Input: part model. Units: mm. Frame: model coordinates. A direction names the side the tool comes from. Coordinates: 2 decimals unless noted, no trailing zeros. Write each loop counter-clockwise with the first axis right and the second up, starting at its lowest first coordinate (ties: lowest second). Pieces come first, ordered by that corner, then holes. Notation, with made-up numbers: M 64.25,67 L 109.25,67 A29 cw 109.25,90 Z; hole C 23.25,74 d9. An arc over 180 degrees is marked long. Write each question's results on one line, items separated by ' | '. Start each with the question number.
1. Pull-direction query (Y, two-part tool) for faces 1 (the flat face through (0.9, -2, 6)), 2 (the flat face through (-1.965, -3.34, -8.381)), 3 (the flat face through (-3.875, 0, -8)); classes: +Y half, -Y half, draft (parallel to the pull), parting line (faces both ways), or undercut.
2. Set-up query: faces 4 (the flat face through (1.91, -3.37, -8.38)), 5 (the cylindrical face through (1.565, -13.017, 6.246)), 6 (the flat face through (2.4, 0, 6)), 7 (the flat face through (-1.91, 3.37, -8.38)). Return all of +Z, -Z, +X, -X, +Y, -Y with unobstructed straight access to the full face (end or side cutting, diameter ignored); none if empty.
3. Section query A-A, the plane y = 0. Output: boundary loops of the cut face in (x, z) (3 decimals).
4. Section query C-C, the plane z = 0.5. Output: boundary loops of the cut face in (x, y), and give its area (3 significant figures).
5. Ray query, probe 1 along Z at (x, y) = (-7, 8.5); probe 2 along Z at (x, y) = (1, 4); probe 3 along X at (y, z) = (0.5, -15) (3 decimals). Return the intervals inside material, ascending.
6. First-contact query: pin 1 (6 mm diameter, centred on x = 11, y = 15.5, fed in from -Z); pin 2 (1.7 mm diameter, centred on y = 1.5, z = 6.5, fed in from +X); pin 3 (10 mm diameter, centred on y = 5, z = -5.5, fed in from -X) (3 decimals). Flat tips, straight axial feed; report the tip coordinate or a pass-through.
7. Section query B-B, the plane z = -11.5. Output: boundary loops of the cut face in (x, y) (3 decimals), and give its area (3 significant figures).
```python
from build123d import *

# Parameters (mm, degrees)
F1_DEPTH  = 17
F2_R      = 4.7
F3_DEPTH  = 6
F4_R      = 19.4
F5_DEPTH  = 3
F6_R      = 1
F7_W      = 1.5
F7_H      = 1.8
F7_W_2    = 1.8
F7_H_2    = 1.5
F8_DEPTH  = 6
F10_DEPTH = 0.5


with BuildPart() as f1:
    # F0 (on Top) → F1 (new body)
    with BuildSketch(Plane.XY):
        Polygon((3.875, -2.2372322931), (3.875, 2.2372322931), (0, 4.4744645862), (-3.875, 2.2372322931), (-3.875, -2.2372322931), (0, -4.4744645862), align=None)
    extrude(amount=-F1_DEPTH)

    # F2 (on face) → F3 (join)
    with BuildSketch(Plane.XY):
        Circle(F2_R)
    extrude(amount=F3_DEPTH)

    # F4 (on face) → F5 (join)
    with BuildSketch(Plane.XY.offset(6)):
        Circle(F4_R)
    extrude(amount=F5_DEPTH)

    # F6
    f6_edges = [f1.edges().sort_by_distance(p)[0] for p in [
        (-19.4, 0, 6),
        (-19.4, 0, 9),
    ]]
    fillet(f6_edges, radius=F6_R)

    # F7 (on face) → F8 (cut)
    with BuildSketch(Plane.XY.offset(9)):
        with Locations((-1.65, 0.05)):
            Rectangle(F7_W, F7_H)
        with Locations((0, 1.7)):
            Rectangle(F7_W_2, F7_H_2)
        with Locations((0, 0.05)):
            Rectangle(F7_W_2, F7_H)
        with Locations((1.65, 0.05)):
            Rectangle(F7_W, F7_H)
        with Locations((0, -1.6)):
            Rectangle(F7_W_2, F7_H_2)
    extrude(amount=-F8_DEPTH, mode=Mode.SUBTRACT)

    # F9 (on face) → F10 (cut)
    with BuildSketch(Plane(origin=(0, 0, 6), x_dir=(1, 0, 0), z_dir=(0, 0, -1))):
        with BuildLine():
            Line((0.12, 16.1495609697), (0.12, 16.3995609697))
            ThreePointArc((0.12, 16.3995609697), (-1.8790989856, 14.4595880123), (0, 12.4031642156))
            Line((0, 12.4031642156), (0, 12.6536801032))
            ThreePointArc((0, 12.6536801032), (-1.6289699135, 14.4595963078), (0.12, 16.1495609697))
        make_face()
        with BuildLine():
            Line((0, 12.6536801032), (0, 12.4031642156))
            ThreePointArc((0, 12.4031642156), (0.1250097944, 12.3995672443), (0.25, 12.4037904418))
            Line((0.25, 12.4037904418), (0.25, 12.6543962211))
            ThreePointArc((0.25, 12.6543962211), (0.1250128042, 12.6495681492), (0, 12.6536801032))
        make_face()
        with BuildLine():
            ThreePointArc((0.25, 12.4037904418), (0.1250097944, 12.3995672443), (0, 12.4031642156))
            Line((0, 12.4031642156), (0, 10.8995609697))
            Line((0, 10.8995609697), (0.25, 10.8995609697))
            Line((0.25, 10.8995609697), (0.25, 12.4037904418))
        make_face()
        with BuildLine():
            Line((0.25, 12.6543962211), (0.25, 12.4037904418))
            ThreePointArc((0.25, 12.4037904418), (1.5794519519, 13.0320815366), (2.12, 14.3995609697))
            Line((2.12, 14.3995609697), (1.87, 14.3995609697))
            ThreePointArc((1.87, 14.3995609697), (1.865506934, 14.2742392103), (1.8520508076, 14.1495609697))
            ThreePointArc((1.8520508076, 14.1495609697), (1.3140216535, 13.1201813189), (0.25, 12.6543962211))
        make_face()
        with BuildLine():
            Line((0, 14.3995609697), (0, 12.6536801032))
            ThreePointArc((0, 12.6536801032), (0.1250128042, 12.6495681492), (0.25, 12.6543962211))
            Line((0.25, 12.6543962211), (0.25, 14.1495609697))
            Line((0.25, 14.1495609697), (1.8520508076, 14.1495609697))
            ThreePointArc((1.8520508076, 14.1495609697), (1.865506934, 14.2742392103), (1.87, 14.3995609697))
            Line((1.87, 14.3995609697), (0, 14.3995609697))
        make_face()
    extrude(amount=-F10_DEPTH, mode=Mode.SUBTRACT)


solid = f1.part
```
Answer:
1) face 1: undercut | face 2: -Y half | face 3: draft
2) face 4: -Z, +X, -Y | face 5: -Z | face 6: +Z | face 7: -Z, -X, +Y
3) outline: M -19.4,7 A1 ccw -18.4,6 L -4.7,6 L -4.7,0 L -3.875,0 L -3.875,-17 L 3.875,-17 L 3.875,0 L 4.7,0 L 4.7,6 L 18.4,6 A1 ccw 19.4,7 L 19.4,8 A1 ccw 18.4,9 L 2.4,9 L 2.4,3 L -2.4,3 L -2.4,9 L -18.4,9 A1 ccw -19.4,8 Z
4) outline: C 0,0 d9.4 | area: 69.4 mm^2
5) probe 1: 6 to 9 | probe 2: 0 to 9 | probe 3: -3.875 to 3.875
6) pin 1: z = 6 | pin 2: x = 19.38 | pin 3: x = -3.875
7) outline: M -3.875,-2.237 L 0,-4.474 L 3.875,-2.237 L 3.875,2.237 L 0,4.474 L -3.875,2.237 Z | area: 52.0 mm^2
